Geometry: final body of the model. Coordinates: model frame, mm. Face numbers are marked on the shaded views. A direction names the side the tool comes from. Give positions to 0.01 mm unless a question says otherwise; leave off trailing zeros. Write each loop counter-clockwise with the first axis right and the second up, starting at its lowest first coordinate (ties: lowest second). Pieces come first, ordered by that corner, then holes. Notation, with made-up numbers: (-7.5, -9) - (45.5, -9) arc R3 cw to (45.5, -4) - close; hole circle Ø7 at (0, -12.75). An arc over 180 degrees is marked (long way). Use CSV: the item, a comma, the result in double quotes. Start each with the question number.
(1) Line query: probe 1 along X at (y, z) = (104.5, 7.75); probe 2 along Z at (x, y) = (130.5, 120); probe 3 along Z at (x, y) = (79, 135). Output: solid intervals per line, ascending. Write a range as [from, to].
(2) First-contact query: pin 1 Ø8.5 at (x, y) = (-129, 118) entering from +Z; pin 2 Ø3 at (y, z) = (120.5, 10) entering from -X; pin 3 Ø3 at (y, z) = (133, 7) entering from +X. Flat tips, straight axial feed; report the tip coordinate or a pass-through.
(3) Section A-A on y = 115.5. Output: boundary loops of the cut face in (x, z).
(4) Reachability of the marked faces 1 and 2 from +Z, -Z, +X, -X, +Y, -Y: full face, straight path, thin tool, end or side. Return the list, or none.
(5) Section B-B on x = -44. Output: boundary loops of the cut face in (y, z) (3 decimals).
from build123d import *

# Parameters (mm, degrees)
ESQUISSE1_W             = 280.5
ESQUISSE1_H             = 40
BOSS_EXTRU_1_DEPTH      = 5
ESQUISSE2_W             = 246.5
ESQUISSE2_H             = 40
BOSS_EXTRU_2_DEPTH      = 10.25
ENL_V_MAT_EXTRU_1_REACH = 265.5


with BuildPart() as part:
    # Esquisse1 → Boss.-Extru.1 (new body)
    with BuildSketch(Plane.XY):
        with Locations((2.164847162, 117.813864629)):
            Rectangle(ESQUISSE1_W, ESQUISSE1_H)
    extrude(amount=BOSS_EXTRU_1_DEPTH)

    # Esquisse2 → Boss.-Extru.2 (add)
    with BuildSketch(Plane.XY.offset(5)):
        with Locations((2.164847162, 117.813864629)):
            Rectangle(ESQUISSE2_W, ESQUISSE2_H)
    extrude(amount=BOSS_EXTRU_2_DEPTH)

    # Esquisse3 → Enlèv. mat.-Extru.1 (cut, up to next)
    with BuildSketch(Plane.ZY.offset(121.085152838), mode=Mode.PRIVATE) as enl_v_mat_extru_1_sk1:
        Polygon((10.125, 137.813864629), (15.25, 137.813864629), (15.25, 132.688864629), align=None)
    enl_v_mat_extru_1_tool1 = extrude(enl_v_mat_extru_1_sk1.sketch, amount=-ENL_V_MAT_EXTRU_1_REACH, mode=Mode.PRIVATE) & part.part
    add(enl_v_mat_extru_1_tool1.solids().sort_by_distance((-121.085153, 136.105531, 13.541667))[0], mode=Mode.SUBTRACT)
    # Esquisse3 → Enlèv. mat.-Extru.1 (cut, up to next)
    with BuildSketch(Plane.ZY.offset(121.085152838), mode=Mode.PRIVATE) as enl_v_mat_extru_1_sk2:
        Polygon((15.25, 97.813864629), (15.25, 102.938864629), (10.125, 97.813864629), align=None)
    enl_v_mat_extru_1_tool2 = extrude(enl_v_mat_extru_1_sk2.sketch, amount=-ENL_V_MAT_EXTRU_1_REACH, mode=Mode.PRIVATE) & part.part
    add(enl_v_mat_extru_1_tool2.solids().sort_by_distance((-121.085153, 99.522198, 13.541667))[0], mode=Mode.SUBTRACT)


solid = part.part
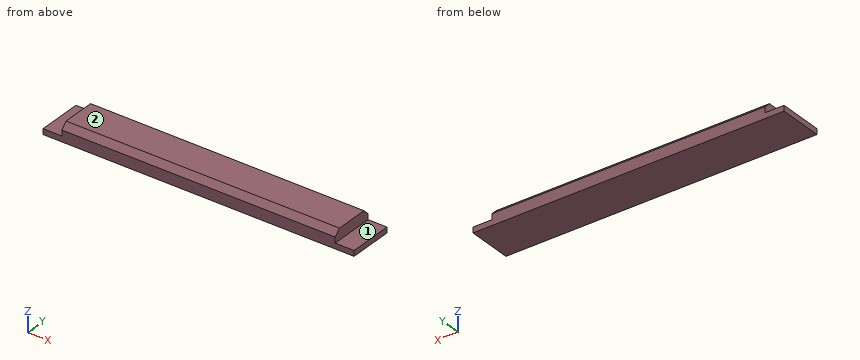
Check values:
1,probe 1,"x = [-121.09, 125.41]"
1,probe 2,"z = [0, 5]"
1,probe 3,"z = [0, 12.94]"
2,pin 1,"stops at z = 5"
2,pin 2,"stops at x = -121.09"
2,pin 3,"stops at x = 125.41"
3,outline,"(-138.09, 0) - (142.41, 0) - (142.41, 5) - (125.41, 5) - (125.41, 15.25) - (-121.09, 15.25) - (-121.09, 5) - (-138.09, 5) - close"
4,face 1,"+Z, +X, +Y, -Y"
4,face 2,"+Z, +X, -X, +Y, -Y"
5,outline,"(97.814, 0) - (137.814, 0) - (137.814, 10.125) - (132.689, 15.25) - (102.939, 15.25) - (97.814, 10.125) - close"
